Could you check a few things on this model? Use its own coordinates, in mm. Face numbers are marked on the shaded views. Coordinates: 2 decimals unless noted, no trailing zeros. Order: outer loops, then holes, each group sorted by start corner. A loop starts at its lowest first (then second) coordinate and runs counter-clockwise, first axis right, second up. Notation, with made-up numbers: (74, 59) - (79, 59) arc R19 ccw to (79, 73) - close; hole circle Ø2 at (-2, -24.5). An arc over 180 degrees is marked (long way). Answer as a JSON object with one key per item and string values. Group by question number.
(1) Will this pin go through, and if not, where does the flat tip stop? P1, Ø11.5, axis at y = 93.85, z = -25, coming from the -X side (1 decimal).
(2) Please list where these lines run through material, in increasing order: probe 1 along Z at (x, y) = (4.5, 93.85); probe 2 along Y at (x, z) = (7.25, -25); probe 3 along Y at (x, z) = (1, -20).
(3) Imagine slicing it at C-C, the plane x = 6. Write out the boundary of the cut face in (y, z), and give its area (3 significant figures).
(4) Imagine slicing it at B-B, the plane z = -25. Write out the boundary of the cut face in (x, y), and give its area (3 significant figures).
(5) Imagine slicing it at A-A, the plane y = 93.85. Write out the boundary of the cut face in (x, z).
(6) We'd pull the mould along Y, two halves only. Please class the marked faces 1, 2 and 3: pulls with the +Y half, pulls with the -Y half, needs draft (parallel to the pull), parting line crosses it, or undercut.
Autodesk Inventor part; units mm, degrees
ref_plane "YZ Plane" through (0, 0, 0) normal (1, 0, 0) x (0, 1, 0)
ref_plane "XZ Plane" through (0, 0, 0) normal (0, 1, 0) x (-1, 0, 0)
ref_plane "XY Plane" through (0, 0, 0) normal (0, 0, 1) x (1, 0, 0)
sketch "Sketch1" plane through (0, 0, 0) normal (1, 0, 0) x (0, 1, 0)
  line L0 (0, 0) -> (149, 0)
  line L1 (149, 0) -> (149, -50)
  line L2 (149, -50) -> (0, -50)
  line L3 (0, -50) -> (0, 0)
  line L4 (0, -25) -> (93.85, -25)
  circle A0 centre (93.85, -25) radius 6.5
  dimension "d0" = 149
  dimension "d1" = 50
  dimension "d2" = 93.85
  dimension "d3" = 13
extrude "Extrusion1" add sketch "Sketch1" along normal blind 10
properties part number "tallwall1"
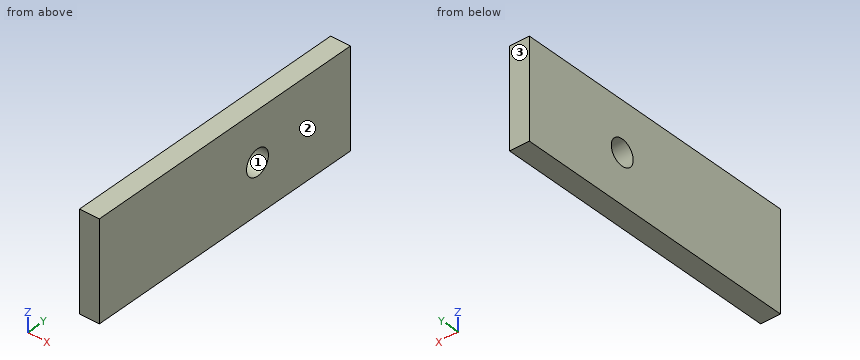
Result set:
{
 "1": {"P1": "passes through"},
 "2": {"probe 1": "z = -50 to -31.5, -18.5 to 0", "probe 2": "y = 0 to 87.35, 100.35 to 149", "probe 3": "y = 0 to 89.7, 98 to 149"},
 "3": {"outline": "(0, -50) - (149, -50) - (149, 0) - (0, 0) - close; hole circle Ø13 at (93.85, -25)", "area": "7,320 mm^2"},
 "4": {"outline": "(0, 0) - (10, 0) - (10, 87.35) - (0, 87.35) - close; (0, 100.35) - (10, 100.35) - (10, 149) - (0, 149) - close", "area": "1,360 mm^2"},
 "5": {"outline": "(0, -50) - (10, -50) - (10, -31.5) - (0, -31.5) - close; (0, -18.5) - (10, -18.5) - (10, 0) - (0, 0) - close"},
 "6": {"face 1": "undercut", "face 2": "needs draft", "face 3": "pulls with the +Y half"}
}
